Autodesk Inventor part; units mm, degrees
ref_plane "YZ Plane" through (0, 0, 0) normal (1, 0, 0) x (0, 1, 0)
ref_plane "XZ Plane" through (0, 0, 0) normal (0, 1, 0) x (-1, 0, 0)
ref_plane "XY Plane" through (0, 0, 0) normal (0, 0, 1) x (1, 0, 0)
sketch "Sketch9" plane through (0, 0, 0) normal (0, 0, 1) x (1, 0, 0)
  line L0 (-54, 0) -> (54, 0)
  line L1 (54, 0) -> (54, -910)
  line L2 (54, -910) -> (-54, -910)
  line L3 (-54, -910) -> (-54, 0)
  point P0 (0, 0)
  point P1 (0, 0)
  dimension "d49" = 108
  dimension "d50" = 910
extrude "Plate4" add sketch "Sketch9" along normal blind 2
sketch "Sketch10" plane through (52.2679, 0, 1) normal (0.8660254, 0, -0.5) x (0, 1, 0)
  line L0 (-910, 0) -> (0, 0)
  line L1 (0, 0) -> (0, 107)
  line L2 (0, 107) -> (-910, 107)
  line L3 (-910, 107) -> (-910, 0)
edge flange "Flange2" height 107 angle 60 thickness 2 bend radius 2 thickness toward (0.8660254, 0, -0.5) relief tear relief width 2 relief depth 1 corner gap 2 corner form 0 edges at (54, -455, 2) (-54, -455, 2) wall of the first edge with corners at (52.2679, -910, 1) (52.2679, 0, 1) (105.7679, 0, 93.6647) (105.7679, -910, 93.6647)
bend "Bend2"
corner "Corner2"
sketch "Sketch11" plane through (0, 0, 2) normal (0, 0, 1) x (1, 0, 0)
  circle A0 centre (0, -53) radius 36
  circle A1 centre (0, -857) radius 36
  line L0 (-51.6906, 0) -> (51.6906, 0)
  line L1 (-51.6906, -910) -> (51.6906, -910)
  line L2 (0, 0) -> (0, -17)
  line L3 (0, -910) -> (0, -893)
  point P0 (0, 0)
  dimension "d62" = 72
  dimension "d68" = 17
  dimension "d69" = 804
extrude "Cut3" cut sketch "Sketch11" against normal blind 2
equation "\"d65\" = Thickness"
equation "\"d51\" = Thickness"
equation "\"d52\" = BendReliefWidth"
equation "\"d53\" = BendReliefDepth"
equation "\"d54\" = MinimumRemnant"
equation "\"d55\" = TransitionRadius"
equation "\"d58\" = BendRadius"
equation "\"d59\" = CornerReliefSize"
equation "\"d60\" = GapSize"
equation "\"d61\" = JacobiRadiusSize"
equation "\"BendRadius\" = Thickness"
equation "\"BendReliefWidth\" = Thickness"
equation "\"BendReliefDepth\" = 0.5 * Thickness"
equation "\"CornerReliefSize\" = 4 * Thickness"
equation "\"MinimumRemnant\" = 2 * Thickness"
equation "\"TransitionRadius\" = BendRadius"
equation "\"JacobiRadiusSize\" = BendRadius"
equation "\"GapSize\" = Thickness"
equation "\"Octaeder_side\" = d41"
equation "\"Octaeder_flange_lenth\" = d42"
properties part number "DSB 122 hex side 1"
Source: CAD feature listing. Evaluate the final solid. Frame: model axes, mm. A direction names the side the tool comes from. Round coordinates to 2 decimals unless told otherwise and drop trailing zeros. Loops run counter-clockwise (first coordinate to the right, second up) from the corner with the lowest first, then second, coordinate; pieces in that order, holes last. Notation, with made-up numbers: (69.25, -32) - (119.25, -32) arc R8 ccw to (119.25, -27) - close; hole circle Ø9 at (47.5, 64.5). An arc over 180 degrees is marked (long way). Write item = value, one per line. Start each with the question number.
(1) Pull-direction query (Y, two-part tool) for faces 1 (the face through (79.23, -448.63, 47.7)), 2 (the face through (-4.686, -821.306, 1.014)); classes: +Y half, -Y half, draft (parallel to the pull), parting line (faces both ways), or undercut.
(2) Ray query, line 1 along Y through (x, z) = (0, 0.55); line 2 along Z through (x, y) = (46.5, -424.5); line 3 along X through (y, z) = (-53, 0.7). Return the intervals inside material, ascending. Write a range as from..to.
(3) Pin query (flat end, axial travel): pin 1 (2 mm diameter, centred on y = -158.5, z = 20, fed in from +X); pin 2 (12 mm diameter, centred on x = 69, y = -675, fed in from -Z); pin 3 (8 mm diameter, centred on y = -592.5, z = 50, fed in from -X). Return the tip coordinate at first contact, or that it passes through.
(4) Section query D-D, the plane y = -760.5. Output: boundary loops of the cut face in (x, z).
(5) Section query B-B, the plane y = -857. Output: boundary loops of the cut face in (x, z), plus the area to 3 significant figures.
(6) Section query C-C, the plane z = 71. Output: boundary loops of the cut face in (x, y).
(7) Section query A-A, the plane x = 0. Output: boundary loops of the cut face in (y, z).
(8) Set-up query: faces 3 (the face through (-79.23, -461.37, 47.7)), 4 (the face through (-81.694, -461.37, 47.967)). Return all of +Z, -Z, +X, -X, +Y, -Y with unobstructed straight access to the full face (end or side cutting, diameter ignored); none if empty.
Conclusion:
q1.face_1 = draft
q1.face_2 = undercut
q2.line_1 = -910..-893, -821..-89, -17..0
q2.line_2 = 0..2
q2.line_3 = -53.95..-36, 36..53.95
q3.pin_1 = 66.12
q3.pin_2 = 15.59
q3.pin_3 = -85.18
q4.outline = (-107.5, 92.66) - (-55.15, 2) arc R4 ccw to (-51.69, 0) - (51.69, 0) arc R4 ccw to (55.15, 2) - (107.5, 92.66) - (105.77, 93.66) - (53.42, 3) arc R2 cw to (51.69, 2) - (-51.69, 2) arc R2 cw to (-53.42, 3) - (-105.77, 93.66) - close
q5.outline = (-107.5, 92.66) - (-55.15, 2) arc R4 ccw to (-51.69, 0) - (-36, 0) - (-36, 2) - (-51.69, 2) arc R2 cw to (-53.42, 3) - (-105.77, 93.66) - close; (36, 0) - (51.69, 0) arc R4 ccw to (55.15, 2) - (107.5, 92.66) - (105.77, 93.66) - (53.42, 3) arc R2 cw to (51.69, 2) - (36, 2) - close
q5.area = 494 mm2
q6.outline = (-94.99, -910) - (-92.68, -910) - (-92.68, 0) - (-94.99, 0) - close; (92.68, -910) - (94.99, -910) - (94.99, 0) - (92.68, 0) - close
q7.outline = (-910, 0) - (-893, 0) - (-893, 2) - (-910, 2) - close; (-821, 0) - (-89, 0) - (-89, 2) - (-821, 2) - close; (-17, 0) - (0, 0) - (0, 2) - (-17, 2) - close
q8.face_3 = +Z, +Y, -Y
q8.face_4 = -Z, -X, +Y, -Y
